from build123d import *

# Parameters (mm, degrees)
SKETCH1_W          = 165.1
SKETCH1_H          = 88.9
EXTRUDE1_DEPTH     = 1.6002
SKETCH2_R          = 2.4384
CUT_EXTRUDE1_DEPTH = 2.6002
SKETCH3_W          = 90.932
SKETCH3_H          = 78.74
EXTRUDE2_DEPTH     = 27.0002


with BuildPart() as part:
    # Sketch1 → Extrude1 (new body)
    with BuildSketch(Plane(origin=(0, 0, 0), x_dir=(1, 0, 0), z_dir=(0, 1, 0))):
        with Locations((82.55, 44.45)):
            Rectangle(SKETCH1_W, SKETCH1_H)
    extrude(amount=EXTRUDE1_DEPTH)

    # Sketch2 → Cut-Extrude1 (cut, through all)
    with BuildSketch(Plane(origin=(0, 1.6002, 0), x_dir=(-1, 0, 0), z_dir=(0, 1, 0))):
        with Locations((-158.75, -6.35)):
            Circle(SKETCH2_R)
        with Locations((-57.15, -6.35)):
            Circle(SKETCH2_R)
        with Locations((-6.35, -6.35)):
            Circle(SKETCH2_R)
        with Locations((-158.75, -82.55)):
            Circle(SKETCH2_R)
        with Locations((-57.15, -82.55)):
            Circle(SKETCH2_R)
        with Locations((-6.35, -82.55)):
            Circle(SKETCH2_R)
    extrude(amount=-CUT_EXTRUDE1_DEPTH, mode=Mode.SUBTRACT)

    # Sketch3 → Extrude2 (add)
    with BuildSketch(Plane.XZ):
        with Locations((107.95, -43.942)):
            Rectangle(SKETCH3_W, SKETCH3_H)
    extrude(amount=EXTRUDE2_DEPTH)


solid = part.part
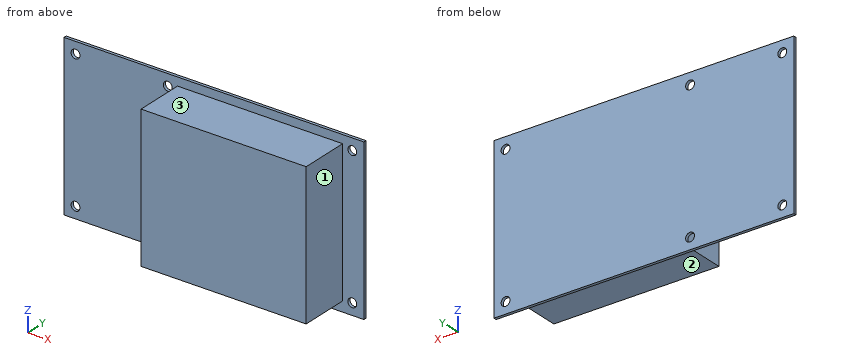
The listing builds one solid part. Answer for the finished solid, in the listing's coordinates (mm). Face numbers are marked on the shaded views. A direction names the side the tool comes from. Give positions to 0.01 mm unless a question says otherwise; leave off trailing zeros. Order: outer loops, then holes, each group sorted by start corner. A loop starts at its lowest first (then second) coordinate and runs counter-clockwise, first axis right, second up. Notation, with made-up numbers: (43.5, 72.5) -> (56.5, 72.5) arc R29 cw to (56.5, 100.5) -> close; hole circle Ø1 at (18, 22.25). An arc over 180 degrees is marked (long way). Put each result on its own line as item: value.
Item 1: A cutting plane is placed at B-B on z = -6.35. Give the vertices of the cut face in (x, y), plus the area to 3 significant figures.
Established:
outline: (0, 0) -> (3.91, 0) -> (3.91, 1.6) -> (0, 1.6) -> close; (8.79, 0) -> (54.71, 0) -> (54.71, 1.6) -> (8.79, 1.6) -> close; (59.59, 0) -> (62.48, 0) -> (62.48, -27) -> (153.42, -27) -> (153.42, 0) -> (156.31, 0) -> (156.31, 1.6) -> (59.59, 1.6) -> close; (161.19, 0) -> (165.1, 0) -> (165.1, 1.6) -> (161.19, 1.6) -> close
area: 2,700 mm^2
Item 2: For the marked faces 1, 2 and 3, determine the directions among +Z, -Z, +X, -X, +Y, -Y from which every point of the face is accessible in a straight line to the end or side of a thin tool.
Established:
face 1: +Z, -Z, +X, -Y
face 2: -Z, +X, -X, -Y
face 3: +Z, +X, -X, -Y
Item 3: A cutting plane is placed at A-A on x = 6.35. Give the vertices of the cut face in (y, z).
Established:
outline: (0, -88.9) -> (1.6, -88.9) -> (1.6, -84.99) -> (0, -84.99) -> close; (0, -80.11) -> (1.6, -80.11) -> (1.6, -8.79) -> (0, -8.79) -> close; (0, -3.91) -> (1.6, -3.91) -> (1.6, 0) -> (0, 0) -> close
Item 4: A cutting plane is placed at C-C on x = 99.5. Give the vertices of the cut face in (y, z).
Established:
outline: (-27, -83.31) -> (0, -83.31) -> (0, -88.9) -> (1.6, -88.9) -> (1.6, 0) -> (0, 0) -> (0, -4.57) -> (-27, -4.57) -> close
Item 5: A cutting plane is placed at D-D on y = -6.75. Give the vertices of the cut face in (x, z).
Established:
outline: (62.48, -83.31) -> (153.42, -83.31) -> (153.42, -4.57) -> (62.48, -4.57) -> close
Item 6: Given P1, Ø13.5, axis at y = -15, z = -51.5, coming from the +X side; P2, Ø13.5, axis at x = 129, y = -8, coming from the +Z side; P3, Ø1, axis at x = 92, y = -17, coming from the -Z side, each flat-ended and moving along its own axis, determine where each tip first touches the part or whether it passes through.
Established:
P1: stops at x = 153.42
P2: stops at z = -4.57
P3: stops at z = -83.31
Item 7: Straight lines are drawn through the part: line 1 (Z direction, x = 158.75, y = 0.55); line 2 (X direction, y = -13, z = -14.5); line 3 (Y direction, x = 9.5, z = -3.5). For each, find the intervals that lie inside material, in ascending order.
Established:
line 1: z = -88.9 to -84.99, -80.11 to -8.79, -3.91 to 0
line 2: x = 62.48 to 153.42
line 3: y = 0 to 1.6
